Can you work these out from the model? Positions are in its coordinate system, mm. A direction names the side the tool comes from. Give positions to 0.01 mm unless a question says otherwise; leave off trailing zeros. Loops run counter-clockwise (first coordinate to the right, second up) from the corner with the lowest first, then second, coordinate; pieces in that order, holes last. Notation, with made-up numbers: (56, 7.25) -> (106, 7.25) arc R33 cw to (106, 38.25) -> close; hole circle Ø9 at (89, 89). An arc over 180 degrees is marked (long way). One line per question, with ' | ' between items.
from build123d import *

# Parameters (mm, degrees)
SKETCH1_R                                       = 0.9
SKETCH1_R_2                                     = 2.575
BOSS_EXTRUDE1_DEPTH                             = 3.05
CSK_FOR_M2_FLAT_HEAD_MACHINE_SCREW1_D           = 1.8
CSK_FOR_M2_FLAT_HEAD_MACHINE_SCREW1_CSINK_D     = 4.4
CSK_FOR_M2_FLAT_HEAD_MACHINE_SCREW1_CSINK_ANGLE = 90


with BuildPart() as part:
    # Sketch1 → Boss-Extrude1 (new body)
    with BuildSketch(Plane.XY):
        with BuildLine():
            Line((12, 0), (12, 6.303908615))
            Line((12, 6.303908615), (4.681585686, 13.62232293))
            Line((4.681585686, 13.62232293), (-0.534038586, 24.807265275))
            ThreePointArc((-0.534038586, 24.807265275), (-8.358318048, 29.755478813), (-9.597116456, 20.581082657))
            Line((-9.597116456, 20.581082657), (0, 0))
            Line((0, 0), (12, 0))
        make_face()
        Polygon((10.727207794, 5.692209589), (8.464466094, 3.429467889), (-0.126881297, 12.02081528), (2.135860402, 14.28355698), align=None, mode=Mode.SUBTRACT)
        with Locations((3.5, 3.5)):
            Circle(SKETCH1_R, mode=Mode.SUBTRACT)
        with Locations((-6.033917608, 24.770785985)):
            Circle(SKETCH1_R_2, mode=Mode.SUBTRACT)
    extrude(amount=BOSS_EXTRUDE1_DEPTH)

    # CSK for M2 Flat Head Machine Screw1 (through all)
    with Locations(Plane.XY.offset(3.05)):
        with Locations((3.5, 3.5)):
            CounterSinkHole(CSK_FOR_M2_FLAT_HEAD_MACHINE_SCREW1_D / 2, CSK_FOR_M2_FLAT_HEAD_MACHINE_SCREW1_CSINK_D / 2, counter_sink_angle=CSK_FOR_M2_FLAT_HEAD_MACHINE_SCREW1_CSINK_ANGLE)


solid = part.part
Q1. On a 3-axis mill with a long thin cutter (end or side, diameter ignored), from which of +Z, -Z, +X, -X, +Y, -Y can I reach the whole of each face in a straight line? I mean faces 4 (the face through (8.392, 9.912, 1.504)), 5 (the face through (0.99, 13.14, 1.5)). Say none if no direction works.
Entries:
face 4: +Z, -Z, +X, +Y | face 5: +Z, -Z
Q2. If we section it at A-A (y = 11.5): Write out the boundary of the cut face in (x, z), plus the area to 3 significant figures.
Entries:
outline: (-5.36, 0) -> (0.39, 0) -> (0.39, 3.05) -> (-5.36, 3.05) -> close; (4.92, 0) -> (6.8, 0) -> (6.8, 3.05) -> (4.92, 3.05) -> close | area: 23.3 mm²
Q3. If we section it at C-C (z = 0.35): Write out the boundary of the cut face in (x, y) (3 decimals).
Entries:
outline: (-9.597, 20.581) -> (0, 0) -> (12, 0) -> (12, 6.304) -> (4.682, 13.622) -> (-0.534, 24.807) arc R5.5 ccw (long way) to start; hole circle Ø5.15 at (-6.034, 24.771); hole (-0.127, 12.021) -> (8.464, 3.429) -> (10.727, 5.692) -> (2.136, 14.284) -> close; hole circle Ø1.8 at (3.5, 3.5)
Q4. For pin 1 Ø4.5 at (x, y) = (-6.03, 24.77) entering from -Z; pin 2 Ø1 at (y, z) = (16.5, 1.5) entering from +X, each with a flat end and sliding along its axis, tell me the tip position at first contact or that it passes through.
Entries:
pin 1: through | pin 2: x = 3.57
Q5. If we mould it in two halves opening along Y, with no side actions, what happens to faces 1 (the face through (12, 3, 2)), 2 (the face through (4.229, 7.665, 1.504)), 3 (the face through (-4.866, 10.435, 1.504))? For each: pulls with the +Y half, pulls with the -Y half, needs draft (parallel to the pull), parting line crosses it, or undercut.
Entries:
face 1: needs draft | face 2: undercut | face 3: pulls with the -Y half
Q6. If we section it at D-D (x = 3.5): Write out the boundary of the cut face in (y, z), plus the area to 3 significant figures.
Entries:
outline: (0, 0) -> (2.6, 0) -> (2.6, 1.75) -> (1.3, 3.05) -> (0, 3.05) -> close; (4.4, 0) -> (8.39, 0) -> (8.39, 3.05) -> (5.7, 3.05) -> (4.4, 1.75) -> close; (12.92, 0) -> (16.16, 0) -> (16.16, 3.05) -> (12.92, 3.05) -> close | area: 28.3 mm²
Q7. If I drill on probe 1 along Y at (x, z) = (3.5, 1.35); probe 2 along Y at (x, z) = (5.75, 1.3); probe 3 along X at (y, z) = (26, 2.3), over which ranges is the centre line in solid material (lowest first)? Write a range as from..to.
Entries:
probe 1: 0..2.6, 4.4..8.39, 12.92..16.16 | probe 2: 0..6.14, 10.67..12.55 | probe 3: -11.39..-8.3, -3.77..-0.67
Q8. If we section it at B-B (x = 6.5): Write out the boundary of the cut face in (y, z).
Entries:
outline: (0, 0) -> (5.39, 0) -> (5.39, 3.05) -> (0, 3.05) -> close; (9.92, 0) -> (11.8, 0) -> (11.8, 3.05) -> (9.92, 3.05) -> close
